Read the model definition and answer for the solid it produces. Units are mm, in the model's axes. A direction names the side the tool comes from. Coordinates: 2 decimals unless noted, no trailing zeros. Loops run counter-clockwise (first coordinate to the right, second up) from the corner with the lowest first, then second, coordinate; pieces in that order, holes last.
Autodesk Fusion 360 part; units mm, degrees
sketch "BaseProfile" plane through (0, 0, 0) normal (0, 1, 0) x (1, 0, 0)
  line L0 (-2.875, 0) -> (2.875, 0)
  line L1 (2.875, 0) -> (2.875, -1)
  line L2 (2.875, -1) -> (4.75, -1)
  line L3 (2.875, -4.25) -> (-2.875, -4.25)
  line L4 (-4.75, -1) -> (-2.875, -1)
  line L5 (-2.875, -1) -> (-2.875, 0)
  line L6 (-4.75, -1) -> (-4.75, -2.75)
  line L7 (-4.75, -2.75) -> (-2.875, -4.25)
  line L8 (4.75, -1) -> (4.75, -2.75)
  line L9 (4.75, -2.75) -> (2.875, -4.25)
  line L10 (0, 7.3711) -> (0, -7.6289)
  dimension "d1" = 5.75
  dimension "d2" = 5.75
  dimension "d3" = 9.5
  dimension "d4" = 1
  dimension "d7" = 1.75
  dimension "d8" = 1.5
extrude "4mmExt" add sketch "BaseProfile" along normal blind 4 makes body 1
extrude "104mmExt" add sketch "BaseProfile" along normal blind 104 separate body makes body 2
extrude "139mmExt" add sketch "BaseProfile" along normal blind 139 separate body makes body 3
extrude "24mmExt" add sketch "BaseProfile" along normal blind 24 separate body makes body 4
extrude "94mmExt (1)" add sketch "BaseProfile" along normal blind 94 separate body makes body 5
sketch "14mm34mm" plane through (0, 0, 0) normal (0, 0, 1) x (1, 0, 0)
  line L0 (-2.875, 15) -> (-2.875, 13)
  arc A0 (-2.875, 13) -> (2.875, 13) centre (0, 13) ccw
  line L1 (2.875, 13) -> (2.875, 15)
  arc A1 (2.875, 15) -> (-2.875, 15) centre (0, 15) ccw
  line L2 (0, 15) -> (0, 13) construction
  line L3 (-2.875, 35) -> (-2.875, 33)
  arc A2 (-2.875, 33) -> (2.875, 33) centre (0, 33) ccw
  line L4 (2.875, 33) -> (2.875, 35)
  arc A3 (2.875, 35) -> (-2.875, 35) centre (0, 35) ccw
  line L5 (0, 35) -> (0, 33) construction
  point P0 (0, 14)
  point P1 (0, 34)
  dimension "d19" = 5.75
  dimension "d20" = 14
  dimension "d21" = 1
  dimension "d42" = 5.75
  dimension "d43" = 20
  dimension "d44" = 1
extrude "14mm34mmCut" cut sketch "14mm34mm" along normal through all bodies 5
extrude "Extrude7" add sketch "BaseProfile" along normal blind 119 separate body makes body 6
sketch "29mm49mm" plane through (0, 0, 0) normal (0, 0, 1) x (1, 0, 0)
  line L0 (-2.875, 30) -> (-2.875, 28)
  arc A0 (-2.875, 28) -> (2.875, 28) centre (0, 28) ccw
  line L1 (2.875, 28) -> (2.875, 30)
  arc A1 (2.875, 30) -> (-2.875, 30) centre (0, 30) ccw
  line L2 (0, 30) -> (0, 28) construction
  line L3 (-2.875, 50) -> (-2.875, 48)
  arc A2 (-2.875, 48) -> (2.875, 48) centre (0, 48) ccw
  line L4 (2.875, 48) -> (2.875, 50)
  arc A3 (2.875, 50) -> (-2.875, 50) centre (0, 50) ccw
  line L5 (0, 50) -> (0, 48) construction
  point P0 (0, 29)
  point P1 (0, 49)
  dimension "d27" = 5.75
  dimension "d28" = 1
  dimension "d29" = 29
  dimension "d30" = 5.75
  dimension "d31" = 20
  dimension "d32" = 1
extrude "29mm49mmCut" cut sketch "29mm49mm" along normal through all bodies 6
extrude "23mmExt" add sketch "BaseProfile" along normal blind 24 separate body makes body 7
sketch "14mm" plane through (0, 0, 0) normal (0, 0, 1) x (1, 0, 0)
  line L0 (-2.875, 15) -> (-2.875, 13)
  arc A0 (-2.875, 13) -> (2.875, 13) centre (0, 13) ccw
  line L1 (2.875, 13) -> (2.875, 15)
  arc A1 (2.875, 15) -> (-2.875, 15) centre (0, 15) ccw
  line L2 (0, 15) -> (0, 13) construction
  point P0 (0, 14)
  dimension "d36" = 5.75
  dimension "d37" = 1
  dimension "d38" = 14
extrude "14mmCut" cut sketch "14mm" along normal through all bodies 7
extrude "94mmExt" add sketch "BaseProfile" along normal blind 94 separate body makes body 8
hidden bodies 1 2 3 4 5 7 8
equation "d8 = 3.25 mm - 1.75 mm"
Item 1: A cutting plane is placed at A-A on y = 98.5. Determine the outline of the cut face in (x, z) (3 decimals).
Numbers:
outline: (-4.75, 1) - (-2.875, 1) - (-2.875, 0) - (2.875, 0) - (2.875, 1) - (4.75, 1) - (4.75, 2.75) - (2.875, 4.25) - (-2.875, 4.25) - (-4.75, 2.75) - close
Item 2: Which of the six approach directions +Z, -Z, +X, -X, +Y, -Y give full straight-line access (tool end or side, diameter ignored) to faces 1 (the face through (-2.875, 29, 3)), 2 (the face through (-4, 59, 1)), 3 (the face through (4, 59, 1))?
Numbers:
face 1: +Z, -Z
face 2: -Z, -X, +Y, -Y
face 3: -Z, +X, +Y, -Y
Item 3: Given pin 1 (2 mm diameter, centred on x = 4, y = 75.5, fed in from -Z); pin 2 (0.5 mm diameter, centred on y = 84.5, z = 0.5, fed in from -X) (3 decimals); pin 3 (2 mm diameter, centred on y = 29, z = 3.5, fed in from -X); pin 4 (0.5 mm diameter, centred on y = 16.5, z = 0.5, fed in from +X) (3 decimals), each flat-ended and moving along its own axis, determine where each tip first touches the part or whether it passes through.
Numbers:
pin 1: stops at z = 1
pin 2: stops at x = -2.875
pin 3: stops at x = -4.75
pin 4: stops at x = 2.875
Item 4: Find the intervals of material crossed by line 1 along Y through (x, z) = (0, 1.4) (3 decimals); line 2 along Y through (x, z) = (-1.5, 3.1); line 3 along Z through (x, y) = (4.5, 84), in increasing order.
Numbers:
line 1: y = 0 to 25.125, 32.875 to 45.125, 52.875 to 119
line 2: y = 0 to 25.55, 32.45 to 45.55, 52.45 to 119
line 3: z = 1 to 2.95
